Here's how the part is built. I have some questions about the finished solid (model axes, mm). A direction names the side the tool comes from. Give positions to 0.01 mm unless a question says otherwise; leave off trailing zeros. Write each loop counter-clockwise with the first axis right and the second up, starting at its lowest first coordinate (ties: lowest second). Pieces come first, ordered by that corner, then holes. Notation, with made-up numbers: (2, 39) -> (46, 39) arc R29 ccw to (46, 66) -> close; hole circle Ø10 at (-34.75, 74). An arc over 180 degrees is marked (long way). Return JSON: item names as keys, results as strings.
from build123d import *

# Parameters (mm, degrees)
SKETCH1_W           = 22.4
SKETCH1_H           = 45.5
BOSS_EXTRUDE1_DEPTH = 1.8
BOSS_EXTRUDE2_START = -1.8
SKETCH2_W           = 14
SKETCH2_H           = 14
BOSS_EXTRUDE2_DEPTH = 8
SKETCH3_W           = 7.4
SKETCH3_H           = 2.6
BOSS_EXTRUDE3_DEPTH = 2.7
SKETCH4_W           = 0.65
SKETCH4_H           = 0.65
BOSS_EXTRUDE4_DEPTH = 5.8
SKETCH6_W           = 9.867
SKETCH6_H           = 2.6
BOSS_EXTRUDE5_DEPTH = 2.7
SKETCH7_W           = 0.65
SKETCH7_H           = 0.65
BOSS_EXTRUDE6_DEPTH = 5.8
FILLET1_R           = 0.5
CHAMFER1_SIZE       = 0.25


with BuildPart() as part:
    # Sketch1 → Boss-Extrude1 (new body)
    with BuildSketch(Plane(origin=(0, 0, 0), x_dir=(1, 0, 0), z_dir=(0, 1, 0))):
        Rectangle(SKETCH1_W, SKETCH1_H)
    extrude(amount=BOSS_EXTRUDE1_DEPTH)

    # Sketch2 → Boss-Extrude2 (add)
    with BuildSketch(Plane(origin=(0, 1.8, 0), x_dir=(1, 0, 0), z_dir=(0, 1, 0)).offset(BOSS_EXTRUDE2_START)):
        with Locations((1.3, -1.25)):
            Rectangle(SKETCH2_W, SKETCH2_H)
    extrude(amount=BOSS_EXTRUDE2_DEPTH)

    # Sketch3 → Boss-Extrude3 (add)
    with BuildSketch(Plane.XY.offset(22.75)):
        with Locations((-6.9, 1.9)):
            Rectangle(SKETCH3_W, SKETCH3_H)
    extrude(amount=BOSS_EXTRUDE3_DEPTH)

    # Sketch4 → Boss-Extrude4 (add)
    with BuildSketch(Plane.XY.offset(25.45)):
        with Locations((-9.366666667, 1.9)):
            Rectangle(SKETCH4_W, SKETCH4_H)
        with Locations((-6.9, 1.9)):
            Rectangle(SKETCH4_W, SKETCH4_H)
        with Locations((-4.433333333, 1.9)):
            Rectangle(SKETCH4_W, SKETCH4_H)
    extrude(amount=BOSS_EXTRUDE4_DEPTH)

    # Sketch6 → Boss-Extrude5 (add)
    with BuildSketch(Plane(origin=(0, 0, -22.75), x_dir=(-1, 0, 0), z_dir=(0, 0, -1))):
        with Locations((5.6665, 1.9)):
            Rectangle(SKETCH6_W, SKETCH6_H)
    extrude(amount=BOSS_EXTRUDE5_DEPTH)

    # Sketch7 → Boss-Extrude6 (add)
    with BuildSketch(Plane(origin=(0, 0, -25.45), x_dir=(-1, 0, 0), z_dir=(0, 0, -1))):
        with Locations((1.966375, 1.9)):
            Rectangle(SKETCH7_W, SKETCH7_H)
        with Locations((4.433125, 1.9)):
            Rectangle(SKETCH7_W, SKETCH7_H)
        with Locations((6.899875, 1.9)):
            Rectangle(SKETCH7_W, SKETCH7_H)
        with Locations((9.366625, 1.9)):
            Rectangle(SKETCH7_W, SKETCH7_H)
    extrude(amount=BOSS_EXTRUDE6_DEPTH)

    # Fillet1
    fillet1_edges = [part.edges().sort_by_distance(p)[0] for p in [
        (8.3, 4.9, 8.25),
        (8.3, 4.9, -5.75),
        (-5.7, 4.9, -5.75),
        (-5.7, 4.9, 8.25),
    ]]
    fillet(fillet1_edges, radius=FILLET1_R)

    # Chamfer1
    chamfer1_edges = [part.edges().sort_by_distance(p)[0] for p in [
        (-5.7, 8, 1.25),
        (1.3, 8, -5.75),
        (8.3, 8, 1.25),
        (1.3, 8, 8.25),
        (-5.553553391, 8, 8.103553391),
        (8.153553391, 8, 8.103553391),
        (8.153553391, 8, -5.603553391),
        (-5.553553391, 8, -5.603553391),
    ]]
    chamfer(chamfer1_edges, length=CHAMFER1_SIZE)


solid = part.part
1. Suppose I cut it at C-C, the plane z = -1. List the corners of the cut face in (x, y) for me.
Taken from the geometry:
{"outline": "(-11.2, 0) -> (11.2, 0) -> (11.2, 1.8) -> (8.3, 1.8) -> (8.3, 7.75) -> (8.05, 8) -> (-5.45, 8) -> (-5.7, 7.75) -> (-5.7, 1.8) -> (-11.2, 1.8) -> close"}
2. Suppose I cut it at A-A, the plane z = -27. List the corners of the cut face in (x, y) for me (3 decimals), and give its area (3 significant figures).
Taken from the geometry:
{"outline": "(-9.692, 1.575) -> (-9.042, 1.575) -> (-9.042, 2.225) -> (-9.692, 2.225) -> close; (-7.225, 1.575) -> (-6.575, 1.575) -> (-6.575, 2.225) -> (-7.225, 2.225) -> close; (-4.758, 1.575) -> (-4.108, 1.575) -> (-4.108, 2.225) -> (-4.758, 2.225) -> close; (-2.291, 1.575) -> (-1.641, 1.575) -> (-1.641, 2.225) -> (-2.291, 2.225) -> close", "area": "1.69 mm²"}
3. Suppose I cut it at D-D, the plane x = 4.75. List the corners of the cut face in (y, z) for me, and give its area (3 significant figures).
Taken from the geometry:
{"outline": "(0, -22.75) -> (1.8, -22.75) -> (1.8, -5.75) -> (7.75, -5.75) -> (8, -5.5) -> (8, 8) -> (7.75, 8.25) -> (1.8, 8.25) -> (1.8, 22.75) -> (0, 22.75) -> close", "area": "169 mm²"}
4. If we mould it in two halves opening along Z, with no side actions, what happens to faces 1 (the face through (-7, 3, 22.75)), 2 (the face through (-3.2, 2, 24))? For each: released by +Z, released by -Z, zero draft, split by the parting line, or undercut.
Taken from the geometry:
{"face 1": "undercut", "face 2": "zero draft"}
5. For pin 1 Ø0.7 at (y, z) = (2, -27) entering from +X; pin 2 Ø1.4 at (x, y) = (3, 1) entering from +Z; pin 3 Ø1.3 at (y, z) = (1.5, 24) entering from -X, each with a flat end and sliding along its axis, tell me the tip position at first contact or that it passes through.
Taken from the geometry:
{"pin 1": "stops at x = -1.64", "pin 2": "stops at z = 22.75", "pin 3": "stops at x = -10.6"}
6. If I drill on line 1 (Z direction, x = -3.25, y = 2); line 2 (Z direction, x = -6, y = 2.75); line 3 (Z direction, x = 3.5, y = 1), over which ranges is the centre line in solid material (lowest first)? Write a range as [from, to].
Taken from the geometry:
{"line 1": "z = [-25.45, -22.75], [-5.75, 8.25], [22.75, 25.45]", "line 2": "z = [-25.45, -22.75], [22.75, 25.45]", "line 3": "z = [-22.75, 22.75]"}
7. Which directions (+Z, -Z, +X, -X, +Y, -Y) give clear straight access to the entire face, cutting with the end or side of a thin tool? Please do faces 3 (the face through (-10.6, 2, -24)), 4 (the face through (-6, 3, -22.75)), 5 (the face through (-10.6, 2, 24)), 6 (the face through (-0.733, 2, -24)).
Taken from the geometry:
{"face 3": "-Z, -X, +Y, -Y", "face 4": "+X, -X, +Y", "face 5": "+Z, -X, +Y, -Y", "face 6": "-Z, +X, +Y, -Y"}
8. Suppose I cut it at B-B, the plane y = 4.5. List the corners of the cut face in (x, z) for me, and give its area (3 significant figures).
Taken from the geometry:
{"outline": "(-5.7, -5.25) arc R0.5 ccw to (-5.2, -5.75) -> (7.8, -5.75) arc R0.5 ccw to (8.3, -5.25) -> (8.3, 7.75) arc R0.5 ccw to (7.8, 8.25) -> (-5.2, 8.25) arc R0.5 ccw to (-5.7, 7.75) -> close", "area": "196 mm²"}
